```python
from build123d import *

# Parameters (mm, degrees)
F0_W          = 50
F0_H          = 100
F0_R          = 8.5
F0_R_2        = 5
F0_R_3        = 3.25
F1_DEPTH      = 150
F2_DEPTH      = 100
F3_DEPTH      = 70
F4_DEPTH      = 130
F8_R          = 7.5
F9_DEPTH      = 15
F10_S5_R      = 5
F10_T6_DEPTH  = 12
F10_S11_R     = 5
F10_T12_DEPTH = 12
F10_S17_R     = 5
F10_T18_DEPTH = 12
F11_SIZE      = 8.5


# Not quite as in the source:
# - a fillet or chamfer that OpenCascade refuses, or shapes differently, is made with other operations: its cross-section is extruded or revolved along the edge and cut away or added


with BuildPart() as f1:
    # F0 (on Top) → F1 (new body)
    with BuildSketch(Plane.XY):
        with Locations((25, 50)):
            Rectangle(F0_W, F0_H)
        with Locations((20, 20)):
            Circle(F0_R, mode=Mode.SUBTRACT)
        with Locations((20, 45)):
            Circle(F0_R, mode=Mode.SUBTRACT)
        with Locations((40, 20)):
            Circle(F0_R_2, mode=Mode.SUBTRACT)
        with Locations((40, 45)):
            Circle(F0_R_2, mode=Mode.SUBTRACT)
        with Locations((20, 70)):
            Circle(F0_R, mode=Mode.SUBTRACT)
        with Locations((12.5, 90)):
            Circle(F0_R_3, mode=Mode.SUBTRACT)
        with Locations((40, 70)):
            Circle(F0_R_2, mode=Mode.SUBTRACT)
        with Locations((25, 90)):
            Circle(F0_R_3, mode=Mode.SUBTRACT)
        with Locations((37.5, 90)):
            Circle(F0_R_3, mode=Mode.SUBTRACT)
        with Locations((12.5, 90)):
            Circle(F0_R_3)
        with Locations((25, 90)):
            Circle(F0_R_3)
        with Locations((37.5, 90)):
            Circle(F0_R_3)
        with Locations((40, 70)):
            Circle(F0_R_2)
        with Locations((20, 70)):
            Circle(F0_R)
        with Locations((40, 45)):
            Circle(F0_R_2)
        with Locations((40, 20)):
            Circle(F0_R_2)
        with Locations((20, 20)):
            Circle(F0_R)
        with Locations((20, 45)):
            Circle(F0_R)
    extrude(amount=F1_DEPTH)

    # F0 (on Top) → F2 (cut)
    with BuildSketch(Plane.XY):
        with Locations((20, 20)):
            Circle(F0_R)
        with Locations((20, 45)):
            Circle(F0_R)
        with Locations((20, 70)):
            Circle(F0_R)
    extrude(amount=F2_DEPTH, mode=Mode.SUBTRACT)

    # F0 (on Top) → F3 (cut)
    with BuildSketch(Plane.XY):
        with Locations((37.5, 90)):
            Circle(F0_R_3)
        with Locations((25, 90)):
            Circle(F0_R_3)
        with Locations((12.5, 90)):
            Circle(F0_R_3)
    extrude(amount=F3_DEPTH, mode=Mode.SUBTRACT)

    # F0 (on Top) → F4 (cut)
    with BuildSketch(Plane.XY):
        with Locations((40, 20)):
            Circle(F0_R_2)
        with Locations((40, 45)):
            Circle(F0_R_2)
        with Locations((40, 70)):
            Circle(F0_R_2)
    extrude(amount=F4_DEPTH, mode=Mode.SUBTRACT)

    # F8 (on 3pt) → F9 (cut, symmetric)
    with BuildSketch(Plane.XY.offset(130)):
        with Locations((40, 70)):
            Circle(F8_R)
        with Locations((40, 45)):
            Circle(F8_R)
        with Locations((40, 20)):
            Circle(F8_R)
    extrude(amount=F9_DEPTH, both=True, mode=Mode.SUBTRACT)

    # F10: chamfer of 5 on 3 edges, made by hand


with BuildPart() as f10_tool2:
    # F10_s3 → F10_t4 (revolve)
    with BuildSketch(Plane.XZ.offset(-70)):
        Polygon((42.5, 115), (47.5, 120), (47.5, 115), align=None)
    revolve(axis=Axis((40, 70, 115), (0, 0, 1)))

    # F10_s5 → F10_t6 (cut, symmetric)
    with BuildSketch(Plane.XY.offset(117.5)):
        with Locations((40, 70)):
            Circle(F10_S5_R)
    extrude(amount=F10_T6_DEPTH, both=True, mode=Mode.SUBTRACT)


with BuildPart() as f1_1:
    add(f1.part)

    # F10_t1: union F10_tool2
    add(f10_tool2.part)


with BuildPart() as f10_tool8:
    # F10_s9 → F10_t10 (revolve)
    with BuildSketch(Plane.XZ.offset(-45)):
        Polygon((42.5, 115), (47.5, 120), (47.5, 115), align=None)
    revolve(axis=Axis((40, 45, 115), (0, 0, 1)))

    # F10_s11 → F10_t12 (cut, symmetric)
    with BuildSketch(Plane.XY.offset(117.5)):
        with Locations((40, 45)):
            Circle(F10_S11_R)
    extrude(amount=F10_T12_DEPTH, both=True, mode=Mode.SUBTRACT)


with BuildPart() as f1_2:
    add(f1_1.part)

    # F10_t7: union F10_tool8
    add(f10_tool8.part)


with BuildPart() as f10_tool14:
    # F10_s15 → F10_t16 (revolve)
    with BuildSketch(Plane.XZ.offset(-20)):
        Polygon((42.5, 115), (47.5, 120), (47.5, 115), align=None)
    revolve(axis=Axis((40, 20, 115), (0, 0, 1)))

    # F10_s17 → F10_t18 (cut, symmetric)
    with BuildSketch(Plane.XY.offset(117.5)):
        with Locations((40, 20)):
            Circle(F10_S17_R)
    extrude(amount=F10_T18_DEPTH, both=True, mode=Mode.SUBTRACT)


with BuildPart() as f1_3:
    add(f1_2.part)

    # F10_t13: union F10_tool14
    add(f10_tool14.part)

    # F11
    f11_edges = [f1_3.edges().sort_by_distance(p)[0] for p in [
        (11.5, 70, 100),
        (11.5, 45, 100),
        (11.5, 20, 100),
    ]]
    chamfer(f11_edges, length=F11_SIZE)


solid = f1_3.part
```
Part model, mm, in its own coordinate system. A direction names the side the tool comes from. Coordinates: 2 decimals unless noted, no trailing zeros. Write each loop counter-clockwise with the first axis right and the second up, starting at its lowest first coordinate (ties: lowest second). Pieces come first, ordered by that corner, then holes.
Item 1: Probe line 1 (Y direction, x = 20, z = 51); line 2 (Y direction, x = 40, z = 138); line 3 (X direction, y = 45, z = 115). List the from-to ranges inside material, lowest first.
Item 2: Mould opens along Z. For faces 1 (the face through (22.126, 69.118, 97.698)), 2 (the face through (40, 70, 145)), 3 (the face through (42.772, 74.348, 117.656)), 4 (the face through (13.255, 14.828, 45.11)) say: released by +Z, released by -Z, zero draft, split by the parting line, or undercut.
Item 3: Slice it at A-A (z = 35.5). Count the separate pieces of the cut face and the enclosed holes in it, and give its area (3 significant figures).
Item 4: Pin check, flat tip, straight feed: pin 1 (2 mm diameter, centred on x = 25.5, y = 91, fed in from -Z). Stop position of the tip, or through.
Item 5: Which spindle directions (+Z, -Z, +X, -X, +Y, -Y) get a long thin tool onto all of the face, cutting with end or side? Do faces 5 (the face through (25, 90, 70)), 6 (the face through (44.92, 46.55, 117.66)), 7 (the face through (30, 51, 0)). Say none if no direction does.
Item 6: Slice it at B-B (z = 87.5). Write the cut outline in (x, y), and give its area (3 significant figures).
Results found:
1. line 1: y = 0 to 11.5, 28.5 to 36.5, 53.5 to 61.5, 78.5 to 100
1. line 2: y = 0 to 12.5, 27.5 to 37.5, 52.5 to 62.5, 77.5 to 100
1. line 3: x = 0 to 35, 45 to 50
2. face 1: released by -Z
2. face 2: undercut
2. face 3: undercut
2. face 4: zero draft
3. separate pieces: 1
3. enclosed holes: 9
3. area: 3,980 mm2
4. pin 1: stops at z = 70
5. face 5: -Z
5. face 6: none
5. face 7: -Z, +X, -X, +Y, -Y
6. outline: (0, 0) - (50, 0) - (50, 100) - (0, 100) - close; hole circle Ø17 at (20, 20); hole circle Ø17 at (20, 45); hole circle Ø17 at (20, 70); hole circle Ø10 at (40, 20); hole circle Ø10 at (40, 45); hole circle Ø10 at (40, 70)
6. area: 4,080 mm2
